Source: three-view drawing plus pictorial views. Frame: mm from the lowest corner of the part. A direction names the side the tool comes from. Round coordinates to 2 decimals unless told otherwise and drop trailing zeros. Order: outer loops, then holes, each group sorted by start corner. A loop starts at its lowest first (then second) coordinate and runs counter-clockwise, first axis right, second up. Notation, with made-up numbers: M 44,-29.75 L 55,-29.75 A16 cw 55,-15.75 Z; hole C -35,69 d4. An arc over 180 degrees is marked long. Return JSON: item names as keys, results as strings. Group by question number.
Q1. Cut plane A-A on z = 10. Output: boundary loops of the cut face in (x, y), and give its area (3 significant figures).
Q2. Access query for the marked faces 1, 2 and 3. Directions: +Z, -Z, +X, -X, +Y, -Y. A direction counts if a zero-diameter tool reaches every point of the face in a straight line with its end or side. Return the directions, or none.
Q3. Contact query for flat-ended pins moving along their axis: pin 1 (3.5 mm diameter, centred on x = 45, z = 25, fed in from -Y); pin 2 (1.6 mm diameter, centred on x = 21.5, y = 9.5, fed in from -Z). Output: stop coordinate, or through.
Q4. Mould query, pull axis Z, two halves, no side actions, for the marked faces 4, 5 and 6. Classes: released by +Z, released by -Z, zero draft, split by the parting line, or undercut.
Q5. Cut plane B-B on x = 45. Output: boundary loops of the cut face in (y, z).
Q6. Ray query, probe 1 along X at (y, z) = (4, 25); probe 2 along X at (y, z) = (1, 26); probe 3 along Z at (x, y) = (10, 9.75). Return the intervals inside material, ascending.
Q7. Cut plane D-D on z = 23. Output: boundary loops of the cut face in (x, y), and give its area (3 significant figures).
Q8. Cut plane C-C on y = 11. Output: boundary loops of the cut face in (x, z), and give its area (3 significant figures).
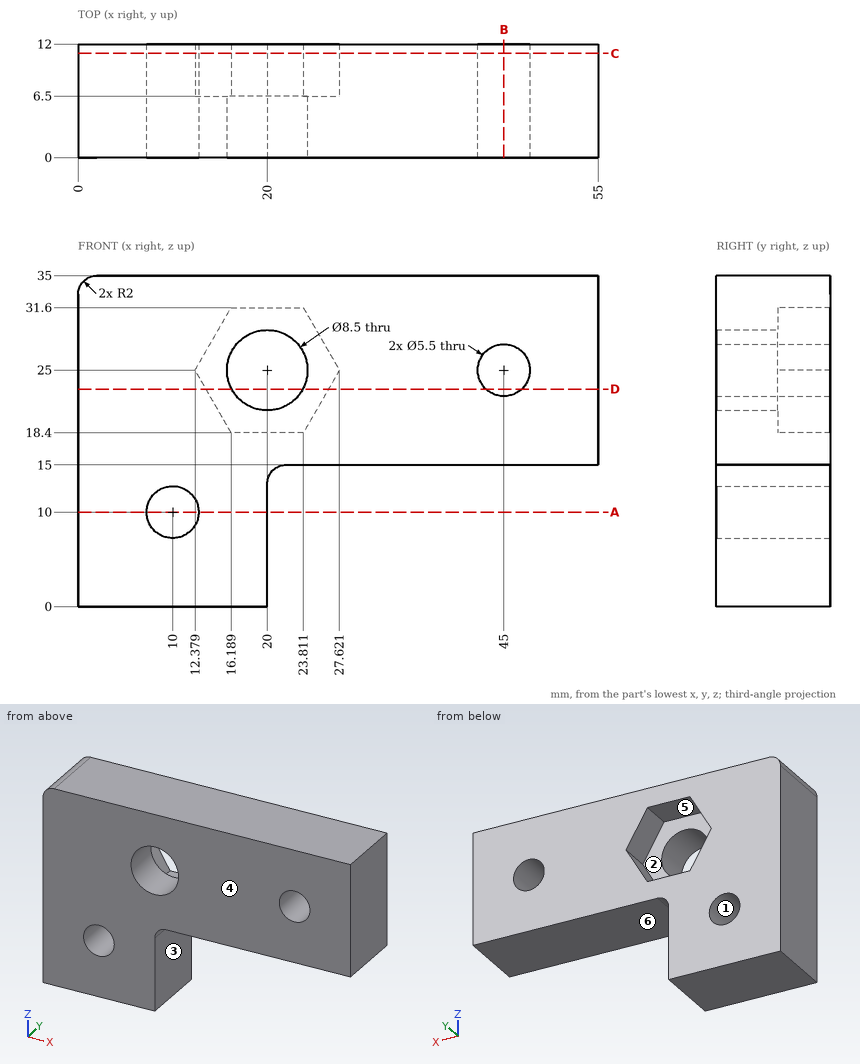
Result sheet:
{
 "1": {"outline": "M 0,0 L 7.25,0 L 7.25,12 L 0,12 Z; M 12.75,0 L 20,0 L 20,12 L 12.75,12 Z", "area": "174 mm²"},
 "2": {"face 1": "+Y, -Y", "face 2": "+Y", "face 3": "-Z, +X, +Y, -Y"},
 "3": {"pin 1": "passes through", "pin 2": "stops at z = 14.52"},
 "4": {"face 4": "zero draft", "face 5": "undercut", "face 6": "released by -Z"},
 "5": {"outline": "M 0,15 L 12,15 L 12,22.25 L 0,22.25 Z; M 0,27.75 L 12,27.75 L 12,35 L 0,35 Z"},
 "6": {"probe 1": "x = 0 to 15.75, 24.25 to 42.25, 47.75 to 55", "probe 2": "x = 0 to 15.87, 24.13 to 42.44, 47.56 to 55", "probe 3": "z = 0 to 7.25, 12.75 to 35"},
 "7": {"outline": "M 0,0 L 16.25,0 L 16.25,6.5 L 13.53,6.5 L 13.53,12 L 0,12 Z; M 23.75,0 L 43.11,0 L 43.11,12 L 26.47,12 L 26.47,6.5 L 23.75,6.5 Z; M 46.89,0 L 55,0 L 55,12 L 46.89,12 Z", "area": "495 mm²"},
 "8": {"outline": "M 0,0 L 20,0 L 20,13 A2 cw 22,15 L 55,15 L 55,35 L 2,35 A2 ccw 0,33 Z; hole C 10,10 d5.5; hole M 12.38,25 L 16.19,18.4 L 23.81,18.4 L 27.62,25 L 23.81,31.6 L 16.19,31.6 Z; hole C 45,25 d5.5", "area": "1,200 mm²"}
}
